Verification items for the finished model (mm, model axes). A direction names the side the tool comes from. Coordinates: 2 decimals unless noted, no trailing zeros. Order: outer loops, then holes, each group sorted by start corner. A loop starts at its lowest first (then second) coordinate and runs counter-clockwise, first axis right, second up. Notation, with made-up numbers: M -12.5,63 L -4.5,63 A27 cw -4.5,82 Z; hole C -23.75,-7 d1. An arc over 180 degrees is marked long. Return JSON: item names as keys, results as strings.
```python
from build123d import *

# Parameters (mm, degrees)
BOSS_EXTRUDE1_DEPTH = 4.7625
SKETCH3_R           = 3.175
CUT_EXTRUDE1_DEPTH  = 4.7625
CUT_EXTRUDE2_DEPTH  = 4.7625
CHAMFER2_SIZE       = 0.635
CHAMFER3_SIZE       = 0.635
CHAMFER4_SIZE       = 0.635
CHAMFER5_SIZE       = 0.635


with BuildPart() as part:
    # Sketch1 → Boss-Extrude1 (new body)
    with BuildSketch(Plane.XY):
        with BuildLine():
            Line((0, 0), (254, 0))
            Line((254, 0), (214.97033738, -156.539426679))
            ThreePointArc((214.97033738, -156.539426679), (203.793912453, -165.003761521), (191.635932139, -158.022289387))
            Line((191.635932139, -158.022289387), (137.120577335, -49.311242034))
            ThreePointArc((137.120577335, -49.311242034), (129.641206804, -41.135892713), (118.984721667, -38.1))
            Line((118.984721667, -38.1), (13.468327891, -38.1))
            ThreePointArc((13.468327891, -38.1), (10.340767596, -37.023094628), (8.539225601, -34.24896323))
            Line((8.539225601, -34.24896323), (0, 0))
        make_face()
    extrude(amount=BOSS_EXTRUDE1_DEPTH)

    # Sketch3 → Cut-Extrude1 (cut)
    with BuildSketch(Plane.XY.offset(4.7625)):
        with Locations((203.2, -152.4)):
            Circle(SKETCH3_R)
        with Locations((203.2, -19.05)):
            Circle(SKETCH3_R)
    extrude(amount=-CUT_EXTRUDE1_DEPTH, mode=Mode.SUBTRACT)

    # Sketch4 → Cut-Extrude2 (cut)
    with BuildSketch(Plane.XY.offset(4.7625)):
        with BuildLine():
            Line((161.039986458, -38.1), (218.365309961, -38.1))
            ThreePointArc((218.365309961, -38.1), (222.368404589, -40.052439705), (223.294412251, -44.40896323))
            Line((223.294412251, -44.40896323), (204.257595645, -120.761464306))
            ThreePointArc((204.257595645, -120.761464306), (199.887371396, -124.581664902), (194.787476915, -121.809685673))
            Line((194.787476915, -121.809685673), (156.498970018, -45.457184596))
            ThreePointArc((156.498970018, -45.457184596), (156.717111388, -40.511826256), (161.039986458, -38.1))
        make_face()
    extrude(amount=-CUT_EXTRUDE2_DEPTH, mode=Mode.SUBTRACT)

    # Chamfer2
    chamfer2_edges = [part.edges().sort_by_distance(p)[0] for p in [
        (200.025, -152.4, 4.7625),
    ]]
    chamfer(chamfer2_edges, length=CHAMFER2_SIZE)

    # Chamfer3
    chamfer3_edges = [part.edges().sort_by_distance(p)[0] for p in [
        (200.025, -19.05, 4.7625),
    ]]
    chamfer(chamfer3_edges, length=CHAMFER3_SIZE)

    # Chamfer4
    chamfer4_edges = [part.edges().sort_by_distance(p)[0] for p in [
        (200.025, -19.05, 0),
    ]]
    chamfer(chamfer4_edges, length=CHAMFER4_SIZE)

    # Chamfer5
    chamfer5_edges = [part.edges().sort_by_distance(p)[0] for p in [
        (200.025, -152.4, 0),
    ]]
    chamfer(chamfer5_edges, length=CHAMFER5_SIZE)


solid = part.part
```
Q1. Cross-section at D-D, the plane x = 31.5. Record the boundary of the cut face in (y, z), and give its area (3 significant figures).
Values:
{"outline": "M -38.1,0 L 0,0 L 0,4.76 L -38.1,4.76 Z", "area": "181 mm^2"}
Q2. Cross-section at B-B, the plane y = -152.4. Record the boundary of the cut face in (x, z) (1 decimal).
Values:
{"outline": "M 188.8,0 L 199.4,0 L 200,0.6 L 200,4.1 L 199.4,4.8 L 188.8,4.8 Z; M 206.4,0.6 L 207,0 L 216,0 L 216,4.8 L 207,4.8 L 206.4,4.1 Z"}
Q3. Tool access check on faces 1 (the face through (234.76, -77.17, 2.35)), 2 (the face through (199.97, -124.57, 2.41)), 3 (the face through (67, -38.1, 2)). Record the directions out of +Z, -Z, +X, -X, +Y, -Y that give a thin tool (end or side, any length) a straight path to the whole face; none if there is none.
Values:
{"face 1": "+Z, -Z, +X, -Y", "face 2": "+Z, -Z", "face 3": "+Z, -Z, -X, -Y"}
Q4. Draft check along Y on faces 4 (the face through (204.7, -155.2, 2.4)), 5 (the face through (125, 0, 2)), 6 (the face through (146, -39, 0)). Enter one of: pulls with the +Y half, pulls with the -Y half, needs draft (parallel to the pull), parting line crosses it, or undercut.
Values:
{"face 4": "undercut", "face 5": "pulls with the +Y half", "face 6": "needs draft"}
Q5. Cross-section at C-C, the plane y = -66. Record the boundary of the cut face in (x, z).
Values:
{"outline": "M 145.49,0 L 166.8,0 L 166.8,4.76 L 145.49,4.76 Z; M 217.91,0 L 237.54,0 L 237.54,4.76 L 217.91,4.76 Z"}
Q6. Cross-section at A-A, the plane z = 1.8. State how many separate pieces and enclosed holes the cut face has, and give its area (3 significant figures).
Values:
{"separate pieces": "1", "enclosed holes": "3", "area": "14,100 mm^2"}
Q7. Material ranges on line 1 along Y through (x, z) = (26, 2.3); line 2 along Y through (x, z) = (203.2, 2.1) (3 decimals); line 3 along Y through (x, z) = (185.5, 2.15), recorded low to high.
Values:
{"line 1": "-38.1 to 0", "line 2": "-165.028 to -155.575, -149.225 to -122.822, -38.1 to -22.225, -15.875 to 0", "line 3": "-145.79 to -103.29, -38.1 to 0"}
Q8. Go/stop test with flat-tipped pins: pin 1 (1.4 mm diameter, centred on x = 61, z = 1.5, fed in from -Y); pin 2 (7.5 mm diameter, centred on x = 203.2, y = -19.05, fed in from -Z); pin 3 (1.5 mm diameter, centred on x = 214.5, z = 2.5, fed in from -Y). Record where each tip stops, or that it passes through.
Values:
{"pin 1": "y = -38.1", "pin 2": "z = 0.06", "pin 3": "y = -159.07"}
